For this review, use the dimensioned drawing (mm, ordinates from the lowest corner) and the shaded views. A direction names the side the tool comes from. Give positions to 0.01 mm unless a question says otherwise; leave off trailing zeros. Order: outer loops, then holes, each group sorted by start corner. A loop starts at its lowest first (then second) coordinate and runs counter-clockwise, first axis right, second up. Notation, with made-up numbers: M 41.5,-8 L 67.5,-8 A8 cw 67.5,-4 Z; hole C 6.5,49 d8. An arc over 180 degrees is marked long. Use CSV: the item, a comma, the result in double quotes. Start each with the question number.
(1) Clearance check with flat-ended pins moving along their axes: P1, Ø1.8, axis at y = 4, z = 21, coming from the -X side; P2, Ø2.5, axis at y = 4, z = 14, coming from the +X side. State where each tip first meets the part, or that it passes through.
(2) Tool access review of the marked faces 4, 5 and 6: name each direction out of +Z, -Z, +X, -X, +Y, -Y from which nothing blocks a thin tool from reaching the whole face with its end or side.
(3) Consider section C-C (z = 5.65). Write out the cut boundary in (x, y).
(4) Wall thickness on L1, parallel to X at y = 3.95, z = 5.65; L2, parallel to Z at x = 30, y = 1.35; L3, parallel to X at y = 3.3, z = 12.5: over which ranges is each line inside the solid? List them lowest first. Write a range as from..to.
(5) Consider section A-A (x = 14.5). Write out the cut boundary in (y, z).
(6) Consider section D-D (x = 30). Write out the cut boundary in (y, z).
(7) Draft analysis for pull direction Z (two halves, no side actions). For the marked faces 1, 2 and 3, state which applies: pulls with the +Z half, pulls with the -Z half, needs draft (parallel to the pull), parting line crosses it, or undercut.
(8) Consider section B-B (y = 3). Give the number of separate pieces and of enclosed holes in the cut face, and give its area (3 significant figures).
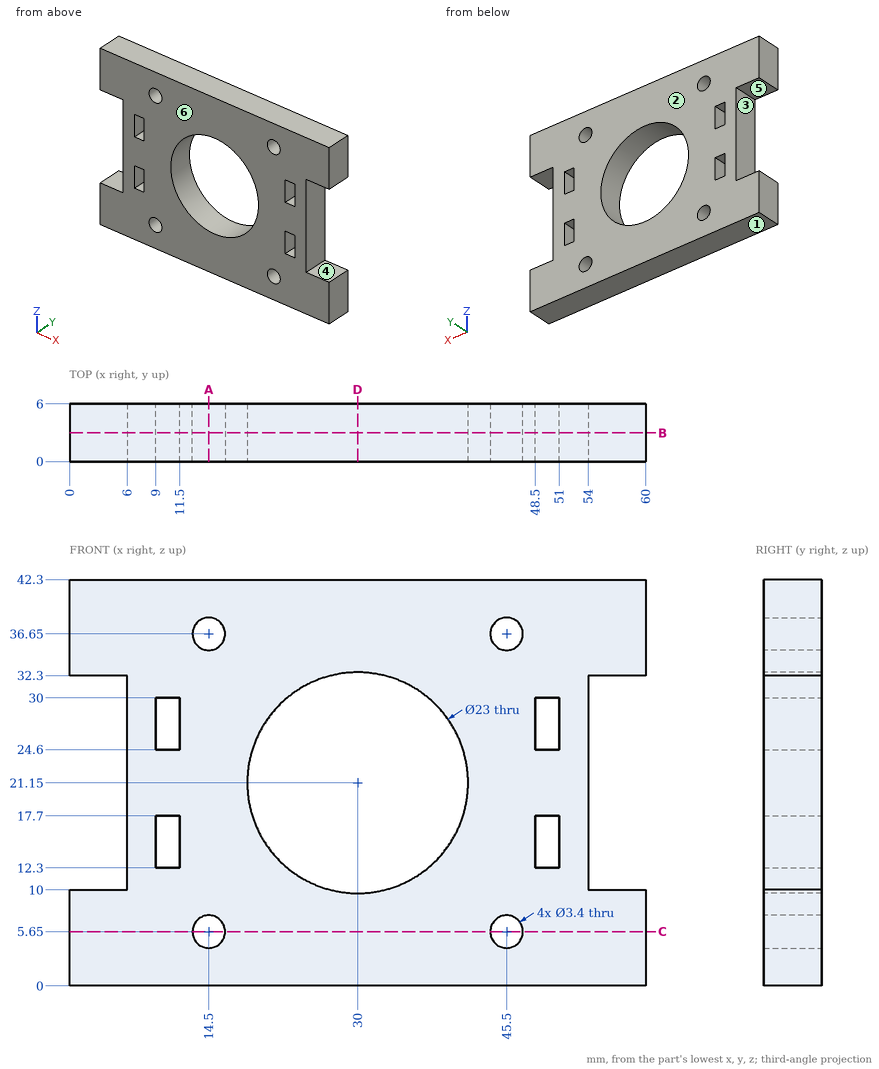
Check result:
1,P1,"stops at x = 6"
1,P2,"stops at x = 54"
2,face 4,"+X, +Y, -Y"
2,face 5,"-X, +Y, -Y"
2,face 6,"+Z, -Z, +X, -X, -Y"
3,outline,"M 0,0 L 12.8,0 L 12.8,6 L 0,6 Z; M 16.2,0 L 43.8,0 L 43.8,6 L 16.2,6 Z; M 47.2,0 L 60,0 L 60,6 L 47.2,6 Z"
4,L1,"x = 0..12.8, 16.2..43.8, 47.2..60"
4,L2,"z = 0..9.65, 32.65..42.3"
4,L3,"x = 6..9, 11.5..22.42, 37.58..48.5, 51..54"
5,outline,"M 0,0 L 6,0 L 6,3.95 L 0,3.95 Z; M 0,7.35 L 6,7.35 L 6,34.95 L 0,34.95 Z; M 0,38.35 L 6,38.35 L 6,42.3 L 0,42.3 Z"
6,outline,"M 0,0 L 6,0 L 6,9.65 L 0,9.65 Z; M 0,32.65 L 6,32.65 L 6,42.3 L 0,42.3 Z"
7,face 1,"pulls with the -Z half"
7,face 2,"needs draft"
7,face 3,"undercut"
8,separate pieces,"1"
8,enclosed holes,"9"
8,area,"1,760 mm^2"
